The listing builds one solid part. Answer for the finished solid, in the listing's coordinates (mm). Give positions to 0.01 mm unless a question says otherwise; leave off trailing zeros. Write each loop counter-clockwise with the first axis right and the second up, starting at its lowest first coordinate (ties: lowest second). Pieces come first, ordered by that corner, then holes. Notation, with made-up numbers: (31.5, 33) - (38.5, 33) arc R23 ccw to (38.5, 64) - close; hole circle Ø4 at (45.5, 82). An arc over 180 degrees is marked (long way). Return JSON: item names as keys, results as strings.
from build123d import *

# Parameters (mm, degrees)
F0_W     = 211.1375
F0_H     = 195.2625
F0_R     = 2.54
F0_W_2   = 109.5375
F0_H_2   = 15.875
F1_DEPTH = 3.175
F2_R     = 19.05
F3_R     = 5.08


with BuildPart() as f1:
    # F0 (on Top) → F1 (new body)
    with BuildSketch(Plane.XY):
        Rectangle(F0_W, F0_H)
        with Locations((0, -76.2)):
            Circle(F0_R, mode=Mode.SUBTRACT)
        with Locations((-15.875, 82.55)):
            Circle(F0_R, mode=Mode.SUBTRACT)
        with Locations((0, 57.94375)):
            Rectangle(F0_W_2, F0_H_2, mode=Mode.SUBTRACT)
        with Locations((15.875, 82.55)):
            Circle(F0_R, mode=Mode.SUBTRACT)
    extrude(amount=F1_DEPTH)

    # F2
    f2_edges = [f1.edges().sort_by_distance(p)[0] for p in [
        (-105.56875, 97.63125, 1.5875),
        (105.56875, 97.63125, 1.5875),
    ]]
    fillet(f2_edges, radius=F2_R)

    # F3
    f3_edges = [f1.edges().sort_by_distance(p)[0] for p in [
        (-54.76875, 50.00625, 1.5875),
        (-54.76875, 65.88125, 1.5875),
        (54.76875, 50.00625, 1.5875),
        (54.76875, 65.88125, 1.5875),
    ]]
    fillet(f3_edges, radius=F3_R)


solid = f1.part
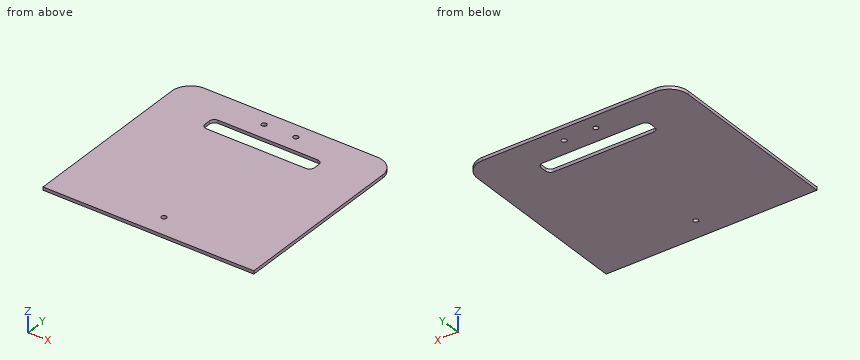
Item 1: A cutting plane is placed at A-A on x = -45.5. Determine the outline of the cut face in (y, z) (3 decimals), then the cut area to 3 significant figures.
Answer below:
{"outline": "(-97.631, 0) - (50.006, 0) - (50.006, 3.175) - (-97.631, 3.175) - close; (65.881, 0) - (97.631, 0) - (97.631, 3.175) - (65.881, 3.175) - close", "area": "570 mm²"}
Item 2: A cutting plane is placed at B-B on y = -76.2. Determine the outline of the cut face in (x, z) (3 decimals), then the cut area to 3 significant figures.
Answer below:
{"outline": "(-105.569, 0) - (-2.54, 0) - (-2.54, 3.175) - (-105.569, 3.175) - close; (2.54, 0) - (105.569, 0) - (105.569, 3.175) - (2.54, 3.175) - close", "area": "654 mm²"}
Item 3: A cutting plane is placed at C-C on x = 0. Determine the outline of the cut face in (y, z) (3 decimals), then the cut area to 3 significant figures.
Answer below:
{"outline": "(-97.631, 0) - (-78.74, 0) - (-78.74, 3.175) - (-97.631, 3.175) - close; (-73.66, 0) - (50.006, 0) - (50.006, 3.175) - (-73.66, 3.175) - close; (65.881, 0) - (97.631, 0) - (97.631, 3.175) - (65.881, 3.175) - close", "area": "553 mm²"}
Item 4: Consider L1, parallel to Y at x = 0, z = 1.4; L2, parallel to Y at x = 49, z = 0.25; L3, parallel to X at y = 79.5, z = 1.4. Determine where each line is inside the solid, lowest interval first.
Answer below:
{"L1": "y = -97.63 to -78.74, -73.66 to 50.01, 65.88 to 97.63", "L2": "y = -97.63 to 50.01, 65.88 to 97.63", "L3": "x = -105.55 to 105.55"}
Item 5: A cutting plane is placed at D-D on z = 1.25. Determine the outline of the cut face in (x, y) (3 decimals), then the cut area to 3 significant figures.
Answer below:
{"outline": "(-105.569, -97.631) - (105.569, -97.631) - (105.569, 78.581) arc R19.05 ccw to (86.519, 97.631) - (-86.519, 97.631) arc R19.05 ccw to (-105.569, 78.581) - close; hole (-54.769, 55.086) arc R5.08 ccw to (-49.689, 50.006) - (49.689, 50.006) arc R5.08 ccw to (54.769, 55.086) - (54.769, 60.801) arc R5.08 ccw to (49.689, 65.881) - (-49.689, 65.881) arc R5.08 ccw to (-54.769, 60.801) - close; hole circle Ø5.08 at (-15.875, 82.55); hole circle Ø5.08 at (0, -76.2); hole circle Ø5.08 at (15.875, 82.55)", "area": "39,300 mm²"}
